Read the model definition and answer for the solid it produces. Units are mm, in the model's axes. Face numbers are marked on the shaded views. A direction names the side the tool comes from. Give positions to 0.01 mm unless a question says otherwise; leave off trailing zeros. Order: outer loops, then holes, each group sorted by start corner. A loop starts at its lowest first (then second) coordinate and runs counter-clockwise, first axis right, second up. Notation, with made-up numbers: (-14.75, 9) -> (34.25, 9) arc R18 ccw to (34.25, 20) -> close; hole circle Ø5 at (-12.5, 65.25). An arc over 180 degrees is marked (long way). Answer as CSV lines item,"result". Start each with the question number.
1) The mould has two halves that part along Y. Classify the marked faces 1, 2, 3 and 4: +Y half, -Y half, draft (parallel to the pull), parting line (faces both ways), or undercut.
2) Find section A-A (y = 20). Determine the outline of the cut face in (x, z).
3) Find section B-B (z = 22). Determine the outline of the cut face in (x, y), and give its area (3 significant figures).
4) Find section D-D (x = 0). State how many separate pieces and enclosed holes the cut face has, and give its area (3 significant figures).
5) Flat-ended cylindrical pins translate along their axes: pin 1 Ø4 at (x, y) = (0, 20) entering from +Z; pin 2 Ø5 at (y, z) = (28.5, 22) entering from +X. Find the tip coordinate at first contact, or state that the pin passes through.
6) Find section C-C (z = -7.5). Determine the outline of the cut face in (x, y).
7) Straight lines are drawn through the part: L1, parallel to Y at x = -3, z = 30; L2, parallel to Y at x = 0, z = 37.7; L3, parallel to X at y = 45, z = 35. For each, find the intervals that lie inside material, in ascending order. Write a range as from..to.
8) For the marked faces 5, 6 and 7, determine the directions among +Z, -Z, +X, -X, +Y, -Y from which every point of the face is accessible in a straight line to the end or side of a thin tool.
```python
from build123d import *

# Parameters (mm, degrees)
ESQUISSE1_W                      = 25
ESQUISSE1_H                      = 15
BOSS_EXTRU_1_DEPTH               = 39
BOSS_EXTRU_1_2_DEPTH             = 39
ESQUISSE3_W                      = 160
ESQUISSE3_H                      = 15
BOSS_EXTRU_2_DEPTH               = 15
ESQUISSE4_R                      = 5
ESQUISSE4_R_2                    = 4
BOSS_EXTRU_5_DEPTH               = 0.8
ESQUISSE4_6_R                    = 4
BOSS_EXTRU_6_DEPTH               = 7.4
CONG_1_R                         = 10
ESQUISSE5_W                      = 11
ESQUISSE5_H                      = 34
ENL_V_MAT_EXTRU_1_DEPTH          = 97.874970968
CONG_2_R                         = 10
ESQUISSE6_R                      = 1.75
ENL_V_MAT_EXTRU_2_DEPTH          = 101.478903258
ESQUISSE11_R                     = 1.75
TROUS_VIS_SUPPORT_CAPTEURS_DEPTH = 97.000052083


with BuildPart() as part:
    # Esquisse1 → Boss.-Extru.1 (new body)
    with BuildSketch(Plane(origin=(0, 0, 0), x_dir=(0, 1, 0), z_dir=(0, 0, 1))):
        with Locations((-45, 0)):
            Rectangle(ESQUISSE1_W, ESQUISSE1_H)
    extrude(amount=BOSS_EXTRU_1_DEPTH)



with BuildPart() as body_2:
    # Esquisse1 → Boss.-Extru.1 2 (new body)
    with BuildSketch(Plane(origin=(0, 0, 0), x_dir=(0, 1, 0), z_dir=(0, 0, 1))):
        with Locations((45, 0)):
            Rectangle(ESQUISSE1_W, ESQUISSE1_H)
    extrude(amount=BOSS_EXTRU_1_2_DEPTH)


with BuildPart() as part_1:
    add(part.part)

    add(body_2.part)  # Boss.-Extru.2 merges body 2
    # Esquisse3 → Boss.-Extru.2 (add)
    with BuildSketch(Plane(origin=(0, 0, 0), x_dir=(0, 1, 0), z_dir=(0, 0, 1))):
        Rectangle(ESQUISSE3_W, ESQUISSE3_H)
    extrude(amount=-BOSS_EXTRU_2_DEPTH)

    # Esquisse4 → Boss.-Extru.5 (add)
    with BuildSketch(Plane(origin=(0, -80, 0), x_dir=(-1, 0, 0), z_dir=(0, -1, 0))):
        with Locations(Location((0, 7.5, 0), (0, 0, 90))):
            Circle(ESQUISSE4_R)
        with Locations(Location((0, 7.5, 0), (0, 0, 90))):
            Circle(ESQUISSE4_R_2, mode=Mode.SUBTRACT)
    boss_extru_5 = extrude(amount=BOSS_EXTRU_5_DEPTH)

    # Esquisse4<6> → Boss.-Extru.6 (add)
    with BuildSketch(Plane(origin=(0, -80, 0), x_dir=(-1, 0, 0), z_dir=(0, -1, 0))):
        with Locations(Location((0, 7.5, 0), (0, 0, 90))):
            Circle(ESQUISSE4_6_R)
    boss_extru_6 = extrude(amount=BOSS_EXTRU_6_DEPTH)

    # Symétrie2: Boss.-Extru.5, Boss.-Extru.6 across plane
    add(boss_extru_5.mirror(Plane.ZX))
    add(boss_extru_6.mirror(Plane.ZX))

    # Congé1
    cong_1_edges = [part_1.edges().sort_by_distance(p)[0] for p in [
        (0, 57.5, 0),
        (0, 32.5, 0),
        (0, -57.5, 0),
        (0, -32.5, 0),
    ]]
    fillet(cong_1_edges, radius=CONG_1_R)

    # Esquisse5 → Enlèv. mat.-Extru.1 (cut, through all)
    with BuildSketch(Plane(origin=(-7.5, 0, 0), x_dir=(0, -1, 0), z_dir=(-1, 0, 0))):
        with Locations((45, 17)):
            Rectangle(ESQUISSE5_W, ESQUISSE5_H)
        with Locations((-45, 17)):
            Rectangle(ESQUISSE5_W, ESQUISSE5_H)
    extrude(amount=-ENL_V_MAT_EXTRU_1_DEPTH, mode=Mode.SUBTRACT)

    # Congé2
    # the kernel refuses this fillet: 10 mm, written as the material it adds along each edge
    with BuildSketch(Plane(origin=(-7.5, 39.5, 0), x_dir=(0, 0, 1), z_dir=(1, 0, 0)), Plane(origin=(-7.5, -39.5, 0), x_dir=(0, -1, 0), z_dir=(1, 0, 0)), Plane(origin=(-7.5, -50.5, 0), x_dir=(0, 0, 1), z_dir=(1, 0, 0))) as cong_2_piece_1:
        with BuildLine():
            CenterArc((CONG_2_R, -CONG_2_R), CONG_2_R, 90, 90)
            Line((0, -CONG_2_R), (0, 0))
            Line((0, 0), (CONG_2_R, 0))
        make_face()
    extrude(amount=15)
    with BuildSketch(Plane(origin=(-7.5, 50.5, 0), x_dir=(0, 0, 1), z_dir=(1, 0, 0))) as cong_2_piece_2:
        with BuildLine():
            CenterArc((CONG_2_R, CONG_2_R), CONG_2_R, 180, 90)
            Line((0, CONG_2_R), (0, 0))
            Line((0, 0), (CONG_2_R, 0))
        make_face()
    extrude(amount=15)

    # Esquisse6 → Enlèv. mat.-Extru.2 (cut, through all)
    with BuildSketch(Plane(origin=(0, 0, 34), x_dir=(1, 0, 0), z_dir=(0, 0, -1))):
        with Locations(Location((0, 45, 0), (0, 0, 180))):
            Circle(ESQUISSE6_R)
        with Locations((0, -45)):
            Circle(ESQUISSE6_R)
    extrude(amount=-ENL_V_MAT_EXTRU_2_DEPTH, mode=Mode.SUBTRACT)

    # Esquisse11 → Trous vis support capteurs (cut, through all)
    with BuildSketch(Plane(origin=(0, 0, 0), x_dir=(0, 1, 0), z_dir=(0, 0, 1))):
        with Locations(Location((20, 0, 0), (0, 0, 270))):
            Circle(ESQUISSE11_R)
        with Locations(Location((-20, 0, 0), (0, 0, 270))):
            Circle(ESQUISSE11_R)
    extrude(amount=-TROUS_VIS_SUPPORT_CAPTEURS_DEPTH, mode=Mode.SUBTRACT)


solid = part_1.part
```
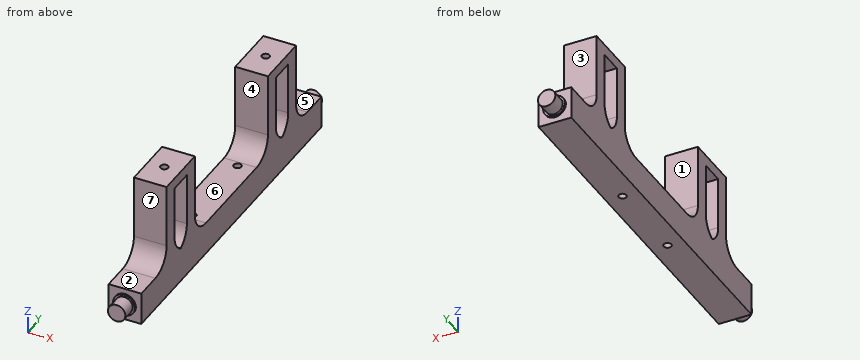
Findings below:
1,face 1,"undercut"
1,face 2,"draft"
1,face 3,"+Y half"
1,face 4,"undercut"
2,outline,"(-7.5, -15) -> (-1.75, -15) -> (-1.75, 0) -> (-7.5, 0) -> close; (1.75, -15) -> (7.5, -15) -> (7.5, 0) -> (1.75, 0) -> close"
3,outline,"(-7.5, -57.5) -> (7.5, -57.5) -> (7.5, -50.5) -> (-7.5, -50.5) -> close; (-7.5, -39.5) -> (7.5, -39.5) -> (7.5, -32.5) -> (-7.5, -32.5) -> close; (-7.5, 32.5) -> (7.5, 32.5) -> (7.5, 39.5) -> (-7.5, 39.5) -> close; (-7.5, 50.5) -> (7.5, 50.5) -> (7.5, 57.5) -> (-7.5, 57.5) -> close"
3,area,"420 mm²"
4,separate pieces,"3"
4,enclosed holes,"0"
4,area,"3,750 mm²"
5,pin 1,"z = 0"
5,pin 2,"through"
6,outline,"(-7.5, -80) -> (-5, -80) -> (-5, -80.8) -> (-4, -80.8) -> (-4, -87.4) -> (4, -87.4) -> (4, -80.8) -> (5, -80.8) -> (5, -80) -> (7.5, -80) -> (7.5, 80) -> (5, 80) -> (5, 80.8) -> (4, 80.8) -> (4, 87.4) -> (-4, 87.4) -> (-4, 80.8) -> (-5, 80.8) -> (-5, 80) -> (-7.5, 80) -> close; hole circle Ø3.5 at (0, -20); hole circle Ø3.5 at (0, 20)"
7,L1,"-57.5..-50.5, -39.5..-32.5, 32.5..39.5, 50.5..57.5"
7,L2,"-57.5..-46.75, -43.25..-32.5, 32.5..43.25, 46.75..57.5"
7,L3,"-7.5..-1.75, 1.75..7.5"
8,face 5,"+Z, +X, -X, +Y"
8,face 6,"+Z, +X, -X"
8,face 7,"+Z, +X, -X, -Y"
